Work out the finished part from the listing and answer in its coordinate system (mm). Face numbers are marked on the shaded views. A direction names the side the tool comes from. Round coordinates to 2 decimals unless told otherwise and drop trailing zeros. Loops run counter-clockwise (first coordinate to the right, second up) from the corner with the lowest first, then second, coordinate; pieces in that order, holes last. Notation, with made-up numbers: (-40, 8) - (-9, 8) arc R10 ccw to (-9, 27) - close; hole circle Ø7 at (8.5, 16.25). An arc over 180 degrees is marked (long way). Use CSV: the item, a comma, the result in double quotes. Start each with the question number.
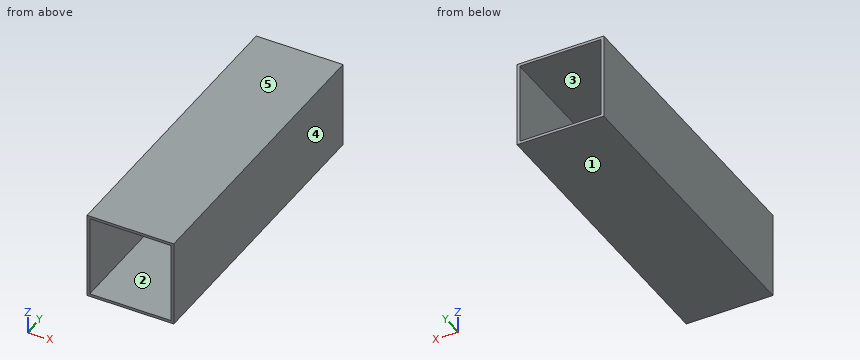
Autodesk Inventor part; units mm, degrees
ref_plane "YZ Plane" through (0, 0, 0) normal (1, 0, 0) x (0, 1, 0)
ref_plane "XZ Plane" through (0, 0, 0) normal (0, 1, 0) x (-1, 0, 0)
ref_plane "XY Plane" through (0, 0, 0) normal (0, 0, 1) x (1, 0, 0)
sketch "Sketch1" plane through (0, 0, 0) normal (0, 1, 0) x (-1, 0, 0)
  line L0 (-50.8, 50.8) -> (-50.8, -50.8)
  line L1 (-50.8, -50.8) -> (50.8, -50.8)
  line L2 (50.8, -50.8) -> (50.8, 50.8)
  line L3 (50.8, 50.8) -> (-50.8, 50.8)
  line L4 (-50.8, 50.8) -> (50.8, -50.8) construction
  line L5 (-50.8, -50.8) -> (50.8, 50.8) construction
  line L6 (-47.625, 47.625) -> (-47.625, -47.625)
  line L7 (-47.625, -47.625) -> (47.625, -47.625)
  line L8 (47.625, -47.625) -> (47.625, 47.625)
  line L9 (47.625, 47.625) -> (-47.625, 47.625)
  line L10 (-47.625, 47.625) -> (47.625, -47.625) construction
  line L11 (-47.625, -47.625) -> (47.625, 47.625) construction
  point P0 (0, 0)
  dimension "d0" = 101.6
  dimension "d1" = 3.175
extrude "Extrusion1" add sketch "Sketch1" along normal blind 355.6
properties part number "AlumPost-4x4xMaxLowBaript" material "Aluminum 6061"
Item 1: The mould has two halves that part along Z. Classify the marked faces 3, 4 and 5: pulls with the +Z half, pulls with the -Z half, needs draft (parallel to the pull), parting line crosses it, or undercut.
Item 2: A cutting plane is placed at A-A (x = 34). Determine the outline of the cut face in (y, z) (3 decimals).
Item 3: A cutting plane is placed at B-B (z = -41). Determine the outline of the cut face in (x, y) (3 decimals).
Item 4: Which of the six approach directions +Z, -Z, +X, -X, +Y, -Y give full straight-line access (tool end or side, diameter ignored) to the marked faces 1 and 2?
Item 5: Find the intervals of material crossed by probe 1 along X at (y, z) = (332.5, -25.5) (3 decimals), in increasing order. Write a range as [from, to].
Item 6: A cutting plane is placed at C-C (y = 328). Determine the outline of the cut face in (x, z) (3 decimals).
Result sheet:
1,face 3,"undercut"
1,face 4,"needs draft"
1,face 5,"pulls with the +Z half"
2,outline,"(0, -50.8) - (355.6, -50.8) - (355.6, -47.625) - (0, -47.625) - close; (0, 47.625) - (355.6, 47.625) - (355.6, 50.8) - (0, 50.8) - close"
3,outline,"(-50.8, 0) - (-47.625, 0) - (-47.625, 355.6) - (-50.8, 355.6) - close; (47.625, 0) - (50.8, 0) - (50.8, 355.6) - (47.625, 355.6) - close"
4,face 1,"-Z, +X, -X, +Y, -Y"
4,face 2,"+Y, -Y"
5,probe 1,"[-50.8, -47.625], [47.625, 50.8]"
6,outline,"(-50.8, -50.8) - (50.8, -50.8) - (50.8, 50.8) - (-50.8, 50.8) - close; hole (-47.625, -47.625) - (47.625, -47.625) - (47.625, 47.625) - (-47.625, 47.625) - close"
